Input: dimensioned drawing with shaded views. Units: mm. Origin: part minimum x, y, z. A direction names the side the tool comes from. Round coordinates to 2 decimals unless told otherwise and drop trailing zeros. Order: outer loops, then holes, each group sorted by start corner. A loop starts at its lowest first (then second) coordinate and runs counter-clockwise, first axis right, second up. Notation, with made-up numbers: (53.25, -7.75) - (87.25, -7.75) arc R26 cw to (87.25, 8.25) - close; hole circle Ø5 at (46.5, -12.75). An arc over 180 degrees is marked (long way). Return JSON: item names as keys, results as strings. Group by question number.
1) Ray query, line 1 (Y direction, x = 37.5, z = 145.5); line 2 (X direction, y = 577, z = 54); line 3 (Z direction, x = 398, y = 265). Return the intervals inside material, ascending. Write a range as from..to.
2) Section C-C, the plane y = 451. Return loops of the section in (x, z), plus the area to 3 significant figures.
3) Contact query for a flat-ended pin moving along its axis: P1, Ø1, axis at x = 227, y = 376.5, coming from the +Z side. Output: stop coordinate, or through.
4) Access query for the marked faces 4 and 5. Directions: +Z, -Z, +X, -X, +Y, -Y. A direction counts if a zero-diameter tool reaches every point of the face in a straight line with its end or side. Return the directions, or none.
5) Section A-A, the plane z = 159.5. Return loops of the section in (x, y).
6) Mould query, pull axis X, two halves, no side actions, for the marked faces 1, 2 and 3. Classes: pulls with the +X half, pulls with the -X half, needs draft (parallel to the pull), parting line crosses it, or undercut.
7) Section B-B, the plane x = 132.5. Return loops of the section in (y, z).
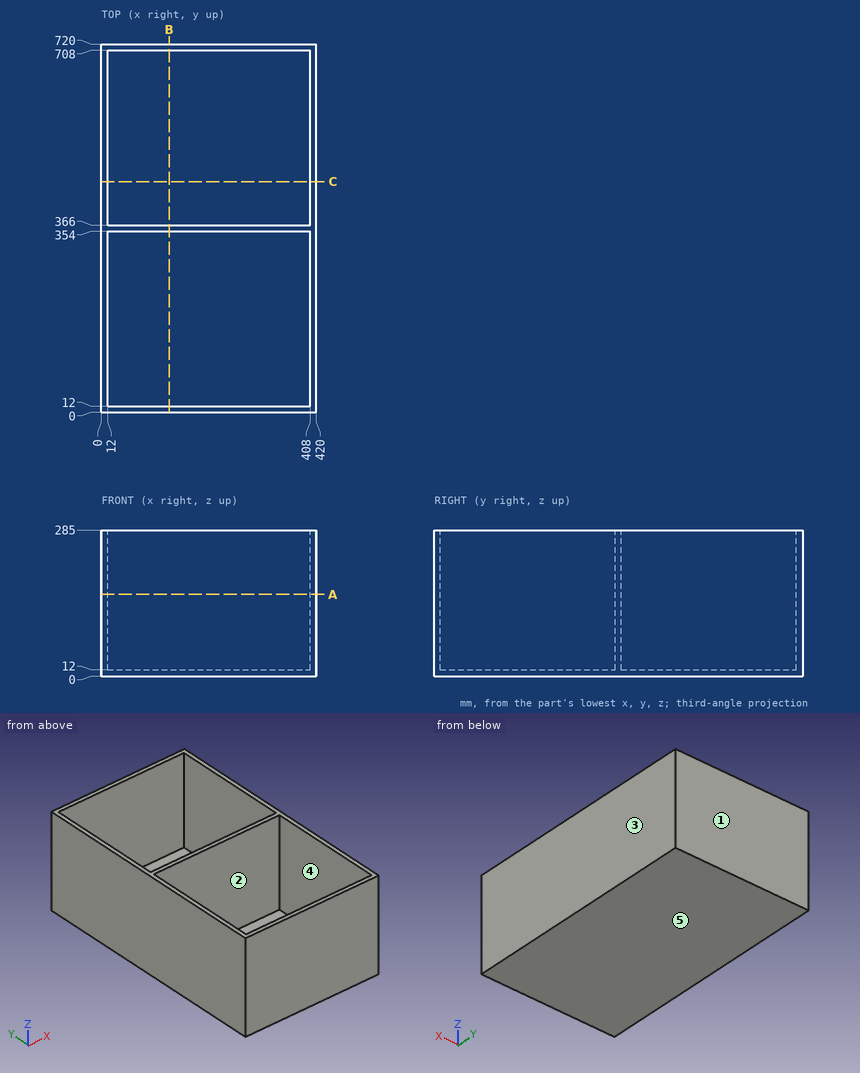
Geometry check:
{
 "1": {"line 1": "0..12, 354..366, 708..720", "line 2": "0..12, 408..420", "line 3": "0..12"},
 "2": {"outline": "(0, 0) - (420, 0) - (420, 285) - (408, 285) - (408, 12) - (12, 12) - (12, 285) - (0, 285) - close", "area": "11,600 mm2"},
 "3": {"P1": "z = 12"},
 "4": {"face 4": "+Z", "face 5": "-Z, +X, -X, +Y, -Y"},
 "5": {"outline": "(0, 0) - (420, 0) - (420, 720) - (0, 720) - close; hole (12, 12) - (408, 12) - (408, 354) - (12, 354) - close; hole (12, 366) - (408, 366) - (408, 708) - (12, 708) - close"},
 "6": {"face 1": "needs draft", "face 2": "undercut", "face 3": "pulls with the +X half"},
 "7": {"outline": "(0, 0) - (720, 0) - (720, 285) - (708, 285) - (708, 12) - (366, 12) - (366, 285) - (354, 285) - (354, 12) - (12, 12) - (12, 285) - (0, 285) - close"}
}
